Could you check a few things on this model? Use its own coordinates, in mm. Give positions to 0.01 mm unless a question says otherwise; leave off trailing zeros. Order: outer loops, then holes, each group sorted by start corner. A loop starts at its lowest first (then second) coordinate and runs counter-clockwise, first axis right, second up. Notation, with made-up numbers: (-29.75, 27.25) - (-11.75, 27.25) arc R25 ccw to (-11.75, 55.25) - close; hole circle Ø4 at (81, 34.5). An arc over 180 degrees is marked (long way). Put each result on its own line as item: value.
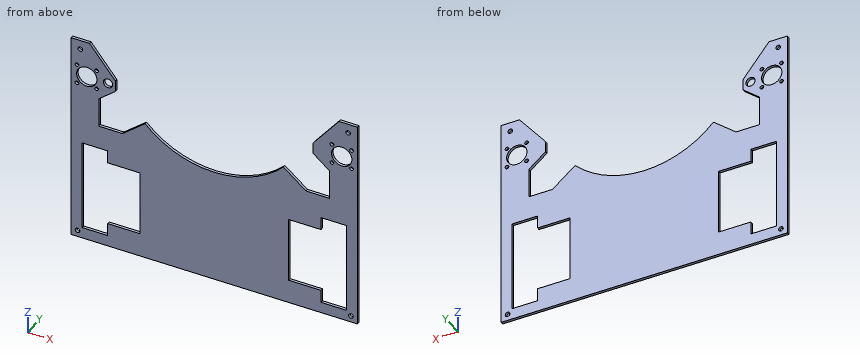
from build123d import *

# Parameters (mm, degrees)
ESQUISSE1_R      = 2.5
ESQUISSE1_R_2    = 11
ESQUISSE1_R_3    = 2
ESQUISSE1_R_4    = 5
EXTRUSION1_DEPTH = 3


with BuildPart() as part:
    # Esquisse1 → Extrusion1 (new body)
    with BuildSketch(Plane(origin=(0, 0, 0), x_dir=(1, 0, 0), z_dir=(0, 1, 0))):
        with BuildLine():
            Line((155, 0), (-155, 0))
            Line((-155, 0), (-155, -230))
            Line((-155, -230), (-135, -230))
            Line((-135, -230), (-107, -195.351767722))
            Line((-107, -195.351767722), (-107, -183.195768703))
            Line((-107, -183.195768703), (-125, -168.649572061))
            Line((-125, -168.649572061), (-125, -136.649572061))
            Line((-125, -136.649572061), (-99.334512084, -136.649572061))
            Line((-99.334512084, -136.649572061), (-74.890281348, -156.403493564))
            ThreePointArc((-74.890281348, -156.403493564), (0, -125), (74.890281348, -156.403493564))
            Line((74.890281348, -156.403493564), (99.334512084, -136.649572061))
            Line((99.334512084, -136.649572061), (125, -136.649572061))
            Line((125, -136.649572061), (125, -168.649572061))
            Line((125, -168.649572061), (107, -183.195768703))
            Line((107, -183.195768703), (107, -195.351767722))
            Line((107, -195.351767722), (135, -230))
            Line((135, -230), (155, -230))
            Line((155, -230), (155, 0))
        make_face()
        with Locations((-148, -7)):
            Circle(ESQUISSE1_R, mode=Mode.SUBTRACT)
        with Locations((148, -7)):
            Circle(ESQUISSE1_R, mode=Mode.SUBTRACT)
        with Locations((-145, -220)):
            Circle(ESQUISSE1_R, mode=Mode.SUBTRACT)
        with Locations((145, -220)):
            Circle(ESQUISSE1_R, mode=Mode.SUBTRACT)
        with Locations((-138, -190)):
            Circle(ESQUISSE1_R_2, mode=Mode.SUBTRACT)
        with Locations((-148.606601718, -179.393398282)):
            Circle(ESQUISSE1_R_3, mode=Mode.SUBTRACT)
        with Locations((-127.393398282, -179.393398282)):
            Circle(ESQUISSE1_R_3, mode=Mode.SUBTRACT)
        with Locations((-127.393398282, -200.606601718)):
            Circle(ESQUISSE1_R_3, mode=Mode.SUBTRACT)
        with Locations((-148.606601718, -200.606601718)):
            Circle(ESQUISSE1_R_3, mode=Mode.SUBTRACT)
        with Locations((138, -190)):
            Circle(ESQUISSE1_R_2, mode=Mode.SUBTRACT)
        with Locations((148.606601718, -200.606601718)):
            Circle(ESQUISSE1_R_3, mode=Mode.SUBTRACT)
        with Locations((127.393398282, -200.606601718)):
            Circle(ESQUISSE1_R_3, mode=Mode.SUBTRACT)
        with Locations((127.393398282, -179.393398282)):
            Circle(ESQUISSE1_R_3, mode=Mode.SUBTRACT)
        with Locations((148.606601718, -179.393398282)):
            Circle(ESQUISSE1_R_3, mode=Mode.SUBTRACT)
        with Locations((-115, -190)):
            Circle(ESQUISSE1_R_4, mode=Mode.SUBTRACT)
        Polygon((-80.5, -26), (-115.5, -26), (-115.5, -12), (-143, -12), (-143, -111), (-115.5, -111), (-115.5, -97), (-80.5, -97), align=None, mode=Mode.SUBTRACT)
        Polygon((115.5, -26), (115.5, -12), (143, -12), (143, -111), (115.5, -111), (115.5, -97), (80.5, -97), (80.5, -26), align=None, mode=Mode.SUBTRACT)
    extrude(amount=EXTRUSION1_DEPTH)


solid = part.part
1) If I drill on line 1 (X direction, y = 0.95, z = 50.5); line 2 (Z direction, x = 138, y = 2.15); line 3 (X direction, y = 0.9, z = 104.5), over which ranges is the centre line in solid material (lowest first)? Write a range as [from, to].
Filled in:
line 1: x = [-155, -143], [-80.5, 80.5], [143, 155]
line 2: z = [0, 12], [111, 179], [201, 230]
line 3: x = [-155, -143], [-115.5, 115.5], [143, 155]
2) I'm going to push a flat-ended pin straight in: pin 1 (17.5 mm diameter, centred on x = 138, z = 190, fed in from -Y). Where does the tip first touch, or does it pass through?
Filled in:
pin 1: passes through
3) Suppose I cut it at D-D, the plane z = 162.5. List the corners of the cut face in (x, y) for me, and give its area (3 significant figures).
Filled in:
outline: (-155, 0) - (-125, 0) - (-125, 3) - (-155, 3) - close; (125, 0) - (155, 0) - (155, 3) - (125, 3) - close
area: 180 mm^2
4) Suppose I cut it at C-C, the plane z = 190. List the corners of the cut face in (x, y) for me, and give its area (3 significant figures).
Filled in:
outline: (-155, 0) - (-149, 0) - (-149, 3) - (-155, 3) - close; (-127, 0) - (-120, 0) - (-120, 3) - (-127, 3) - close; (-110, 0) - (-107, 0) - (-107, 3) - (-110, 3) - close; (107, 0) - (127, 0) - (127, 3) - (107, 3) - close; (149, 0) - (155, 0) - (155, 3) - (149, 3) - close
area: 126 mm^2
5) Suppose I cut it at B-B, the plane x = 96. List the corners of the cut face in (y, z) for me, and give its area (3 significant figures).
Filled in:
outline: (0, 0) - (3, 0) - (3, 26) - (0, 26) - close; (0, 97) - (3, 97) - (3, 139.34) - (0, 139.34) - close
area: 205 mm^2
6) Suppose I cut it at A-A, the plane z = 22.5. List the corners of the cut face in (x, y) for me.
Filled in:
outline: (-155, 0) - (-143, 0) - (-143, 3) - (-155, 3) - close; (-115.5, 0) - (115.5, 0) - (115.5, 3) - (-115.5, 3) - close; (143, 0) - (155, 0) - (155, 3) - (143, 3) - close
